The listing builds one solid part. Answer for the finished solid, in the listing's coordinates (mm). Face numbers are marked on the shaded views. Round coordinates to 2 decimals unless told otherwise and drop trailing zeros. Write each loop counter-clockwise with the first axis right and the second up, starting at its lowest first coordinate (ties: lowest second). Pieces come first, ordered by that corner, then holes. Notation, with made-up numbers: M -38.5,6 L 18.5,6 A20 ccw 18.5,22 Z; hole C 82,81.5 d5. An arc over 180 degrees is marked long. One line per item, written item: value. Start each with the question number.
(1) For a pull along X with two mould halves and no side action, classify the marked faces 1, 2 and 3 as released by +X, released by -X, zero draft, split by the parting line, or undercut.
(2) Section B-B (z = 0.45) is taken. Determine the outline of the cut face in (x, y), plus the area to 3 significant figures.
(3) Given P1, Ø1.5, axis at y = -18, z = 2, coming from the +X side; P2, Ø3, axis at x = -5, y = -9.5, coming from the -Z side, each flat-ended and moving along its own axis, determine where each tip first touches the part or whether it passes through.
(4) Section D-D (x = 42) is taken. Determine the outline of the cut face in (y, z).
(5) Consider probe 1 along Y at (x, z) = (35, 1.55); probe 2 along X at (y, z) = (-11.5, 1.8); probe 3 along Y at (x, z) = (5, 1.9). Determine where each line is inside the solid, lowest interval first.
(6) Section A-A (x = 15) is taken. Determine the outline of the cut face in (y, z).
(7) Section C-C (y = -28) is taken. Determine the outline of the cut face in (x, z), plus the area to 3 significant figures.
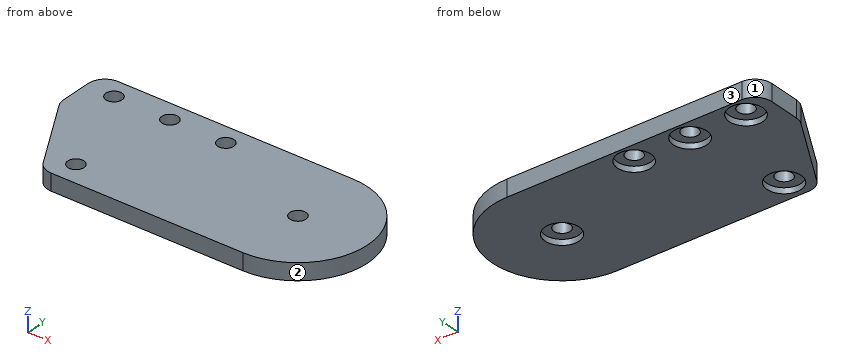
```python
from build123d import *

# Parameters (mm, degrees)
SKETCH_2_R          = 1.45
EXTRUDE_1_DEPTH     = 3
SKETCH_3_R          = 1.45
EXTRUDE_2_DEPTH     = 3
SKETCH_6_R          = 3
CUT_EXTRUDE_2_DEPTH = 1
EXTRUDE_3_DEPTH     = 3
SKETCH_9_R          = 3.05
CUT_EXTRUDE_5_DEPTH = 1
FILLET_1_R          = 3
SKETCH_11_R         = 3.05
CUT_EXTRUDE_7_DEPTH = 1


with BuildPart() as part:
    # 草图2 → 凸台-拉伸1 (new body)
    with BuildSketch(Plane.XY):
        with BuildLine():
            Line((-10, -7), (-10, -16.423561614))
            Line((-10, -16.423561614), (30.724748208, -31.24615776))
            ThreePointArc((30.724748208, -31.24615776), (47.310096913, -21.670602221), (35, -7))
            Line((35, -7), (-10, -7))
        make_face()
        with Locations((35, -19.5)):
            Circle(SKETCH_2_R, mode=Mode.SUBTRACT)
        with Locations((15, -10.5)):
            Circle(SKETCH_2_R, mode=Mode.SUBTRACT)
        with Locations((5, -10.5)):
            Circle(SKETCH_2_R, mode=Mode.SUBTRACT)
        with Locations((-5, -10.5)):
            Circle(SKETCH_2_R, mode=Mode.SUBTRACT)
    extrude(amount=EXTRUDE_1_DEPTH)

    # 草图3 → 凸台-拉伸2 (add)
    with BuildSketch(Plane.XY.offset(3)):
        Polygon((-10, -16.423561614), (32.795912741, -32), (-1.006939105, -32), align=None)
        with Locations((2, -28)):
            Circle(SKETCH_3_R, mode=Mode.SUBTRACT)
    extrude(amount=-EXTRUDE_2_DEPTH)

    # 草图6 → 切除-拉伸2 (cut)
    with BuildSketch(Plane(origin=(0, 0, 0), x_dir=(-1, 0, 0), z_dir=(0, 0, -1))):
        with Locations((-15, -10.5)):
            Circle(SKETCH_6_R)
        with Locations((-5, -10.5)):
            Circle(SKETCH_6_R)
        with Locations((5, -10.5)):
            Circle(SKETCH_6_R)
    extrude(amount=-CUT_EXTRUDE_2_DEPTH, mode=Mode.SUBTRACT)

    # 草图8 → 凸台-拉伸3 (add)
    with BuildSketch(Plane.XY.offset(3)):
        Polygon((32.795912741, -32), (35, -32), (30.724748208, -31.24615776), align=None)
    extrude(amount=-EXTRUDE_3_DEPTH)

    # 草图9 → 切除-拉伸5 (cut)
    with BuildSketch(Plane(origin=(0, 0, 0), x_dir=(-1, 0, 0), z_dir=(0, 0, -1))):
        with Locations((-2, -28)):
            Circle(SKETCH_9_R)
    extrude(amount=-CUT_EXTRUDE_5_DEPTH, mode=Mode.SUBTRACT)

    # 圆角1
    fillet_1_edges = [part.edges().sort_by_distance(p)[0] for p in [
        (-1.006939105, -32, 1.5),
        (-10, -16.423561614, 1.5),
        (-10, -7, 1.5),
    ]]
    fillet(fillet_1_edges, radius=FILLET_1_R)

    # 草图11 → 切除-拉伸7 (cut)
    with BuildSketch(Plane(origin=(0, 0, 0), x_dir=(-1, 0, 0), z_dir=(0, 0, -1))):
        with Locations((-35, -19.5)):
            Circle(SKETCH_11_R)
    extrude(amount=-CUT_EXTRUDE_7_DEPTH, mode=Mode.SUBTRACT)


solid = part.part
```
Recorded:
1. face 1: released by -X
1. face 2: released by +X
1. face 3: zero draft
2. outline: M -10,-15.62 A3 ccw -9.6,-17.12 L -1.87,-30.5 A3 ccw 0.73,-32 L 35,-32 A12.5 ccw 35,-7 L -7,-7 A3 ccw -10,-10 Z; hole C -5,-10.5 d6; hole C 2,-28 d6.1; hole C 5,-10.5 d6; hole C 15,-10.5 d6; hole C 35,-19.5 d6.1
2. area: 1,150 mm2
3. P1: stops at x = 47.48
3. P2: stops at z = 1
4. outline: M -29.86,0 L -9.14,0 L -9.14,3 L -29.86,3 Z
5. probe 1: y = -32 to -20.95, -18.05 to -7
5. probe 2: x = -10 to -6.05, -3.95 to 3.95, 6.05 to 13.95, 16.05 to 44.6
5. probe 3: y = -32 to -11.95, -9.05 to -7
6. outline: M -32,0 L -13.5,0 L -13.5,1 L -11.95,1 L -11.95,3 L -32,3 Z; M -9.05,1 L -7.5,1 L -7.5,0 L -7,0 L -7,3 L -9.05,3 Z
7. outline: M -3.32,0 L -1.05,0 L -1.05,1 L 0.55,1 L 0.55,3 L -3.32,3 Z; M 3.45,1 L 5.05,1 L 5.05,0 L 44.17,0 L 44.17,3 L 3.45,3 Z
7. area: 131 mm2
